Source: CAD feature listing. Evaluate the final solid. Frame: model axes, mm. A direction names the side the tool comes from. Round coordinates to 2 decimals unless told otherwise and drop trailing zeros. Loops run counter-clockwise (first coordinate to the right, second up) from the corner with the lowest first, then second, coordinate; pieces in that order, holes last. Notation, with made-up numbers: (85, -2.5) -> (116, -2.5) arc R15 cw to (116, 4.5) -> close; hole circle Ø4 at (66.25, 88). An arc over 180 degrees is marked (long way). Put each result on its own line as item: value. Start each with the question number.
1. Cut plane D-D (x = -17.5). Return the cut outline in (y, z) (3 decimals), then the cut area to 3 significant figures.
2. Contact query for flat-ended pins moving along their axis: pin 1 (2 mm diameter, centred on x = 15, y = 2, fed in from +Z); pin 2 (0.5 mm diameter, centred on y = 3, z = 6, fed in from -X). Output: stop coordinate, or through.
3. Draft query along X for faces 1 (the cylindrical face through (1.431, 3.131, 4.543)), 2 (the flat face through (0, 0, -6)), 3 (the cylindrical face through (-5.395, 3.131, 8.62)). Return one class per face: pulls with the +X half, pulls with the -X half, needs draft (parallel to the pull), parting line crosses it, or undercut.
4. Cut plane B-B (x = 0). State how many separate pieces and enclosed holes the cut face has, then the cut area to 3 significant figures.
5. Cut plane A-A (z = 0). Return the cut outline in (x, y), then the cut area to 3 significant figures.
6. Material intervals for L1, parallel to X at y = 4.5, z = 0; L2, parallel to Y at x = 0, z = -7.45; L3, parallel to Z at x = 21.5, y = 4.5 (3 decimals), sorted ascending.
7. Set-up query: faces 4 (the flat face through (20, 3, 2.762)), 5 (the cylindrical face through (-0.727, 4.315, -7.08)), 6 (the flat face through (-21, 3, 2.762)). Return all of +Z, -Z, +X, -X, +Y, -Y with unobstructed straight access to the full face (end or side cutting, diameter ignored); none if empty.
```python
from build123d import *

# Parameters (mm, degrees)
SKETCH1_W                  = 63.5
SKETCH1_H                  = 19.05
SKETCH1_R                  = 4.7625
BOSS_EXTRUDE1_DEPTH        = 6.35
F_6_32_TAPPED_HOLE1_REACH  = 39.567
F_6_32_TAPPED_HOLE1_BORE_R = 1.35255
CUT_EXTRUDE1_REACH         = 35.751
SKETCH5_W                  = 25.4
SKETCH5_H                  = 6.7627246
FILLET1_R                  = 3.175


with BuildPart() as part:
    # Sketch1 → Boss-Extrude1 (new body)
    with BuildSketch(Plane(origin=(0, 0, 0), x_dir=(1, 0, 0), z_dir=(0, 1, 0))):
        Rectangle(SKETCH1_W, SKETCH1_H)
        with Locations(Location((0, 0, 0), (0, 0, 270))):
            Circle(SKETCH1_R, mode=Mode.SUBTRACT)
    extrude(amount=BOSS_EXTRUDE1_DEPTH)

    # #6-32 Tapped Hole1 bore → #6-32 Tapped Hole1 (cut, up to next)
    with BuildSketch(Plane(origin=(0, 0, -9.525), x_dir=(-1, 0, 0), z_dir=(0, 0, -1)), mode=Mode.PRIVATE) as f_6_32_tapped_hole1_sk1:
        with Locations((0, 3.175)):
            Circle(F_6_32_TAPPED_HOLE1_BORE_R)
    f_6_32_tapped_hole1_tool1 = extrude(f_6_32_tapped_hole1_sk1.sketch, amount=-F_6_32_TAPPED_HOLE1_REACH, mode=Mode.PRIVATE) & part.part
    add(f_6_32_tapped_hole1_tool1.solids().sort_by_distance((0, 3.175, -9.525))[0], mode=Mode.SUBTRACT)

    # Sketch5 → Cut-Extrude1 (cut, up to next)
    with BuildSketch(Plane(origin=(0, 6.35, 0), x_dir=(1, 0, 0), z_dir=(0, 1, 0)), mode=Mode.PRIVATE) as cut_extrude1_sk1:
        with Locations((19.05, -6.1436377)):
            Rectangle(SKETCH5_W, SKETCH5_H)
    cut_extrude1_tool1 = extrude(cut_extrude1_sk1.sketch, amount=-CUT_EXTRUDE1_REACH, mode=Mode.PRIVATE) & part.part
    # Sketch5 → Cut-Extrude1 (cut, up to next)
    with BuildSketch(Plane(origin=(0, 6.35, 0), x_dir=(1, 0, 0), z_dir=(0, 1, 0)), mode=Mode.PRIVATE) as cut_extrude1_sk2:
        with Locations((-19.05, -6.1436377)):
            Rectangle(SKETCH5_W, SKETCH5_H)
    cut_extrude1_tool2 = extrude(cut_extrude1_sk2.sketch, amount=-CUT_EXTRUDE1_REACH, mode=Mode.PRIVATE) & part.part
    add(cut_extrude1_tool1.solids().sort_by_distance((19.05, 6.35, 6.143638))[0], mode=Mode.SUBTRACT)
    add(cut_extrude1_tool2.solids().sort_by_distance((-19.05, 6.35, 6.143638))[0], mode=Mode.SUBTRACT)

    # Fillet1
    fillet1_edges = [part.edges().sort_by_distance(p)[0] for p in [
        (-6.35, 3.175, 2.7622754),
        (-6.35, 3.175, 9.525),
        (6.35, 3.175, 9.525),
        (6.35, 3.175, 2.7622754),
    ]]
    fillet(fillet1_edges, radius=FILLET1_R)


solid = part.part
```
Solution:
1. outline: (0, -9.525) -> (6.35, -9.525) -> (6.35, 2.762) -> (0, 2.762) -> close
1. area: 78.0 mm^2
2. pin 1: stops at z = 2.76
2. pin 2: stops at x = -6.36
3. face 1: undercut
3. face 2: needs draft
3. face 3: pulls with the -X half
4. separate pieces: 3
4. enclosed holes: 0
4. area: 47.6 mm^2
5. outline: (-31.75, 0) -> (-4.76, 0) -> (-4.76, 6.35) -> (-31.75, 6.35) -> close; (4.76, 0) -> (31.75, 0) -> (31.75, 6.35) -> (4.76, 6.35) -> close
5. area: 343 mm^2
6. L1: x = -31.75 to -4.76, 4.76 to 31.75
6. L2: y = 0 to 1.82, 4.53 to 6.35
6. L3: z = -9.525 to 2.762
7. face 4: +Z, +X, +Y, -Y
7. face 5: -Z
7. face 6: +Z, -X, +Y, -Y
